from build123d import *

# Parameters (mm, degrees)
F0_R     = 75.961814
F0_R_2   = 59.912774
F1_DEPTH = 20.066
F2_R     = 7.541578
F2_R_2   = 7.528696
F2_R_3   = 6.425278
F2_R_4   = 7.130382
F2_R_5   = 7.551866
F2_R_6   = 7.528699
F2_R_7   = 7.576505
F2_R_8   = 7.567783
F3_DEPTH = 20.067
F4_SIZE  = 0.254


with BuildPart() as f1:
    # F0 (on Front) → F1 (new body)
    with BuildSketch(Plane.XZ):
        Circle(F0_R)
        Circle(F0_R_2, mode=Mode.SUBTRACT)
        Circle(F0_R_2)
        with BuildLine():
            ThreePointArc((49.361188, 15.14638), (51.061693, 7.657884), (51.632738, 0))
            ThreePointArc((51.632738, 0), (51.517245, -3.451544), (51.171281, -6.887647))
            ThreePointArc((51.171281, -6.887647), (50.183668, -12.146567), (48.657094, -17.275036))
            ThreePointArc((48.657094, -17.275036), (47.264303, -20.785219), (45.618675, -24.184213))
            ThreePointArc((45.618675, -24.184213), (40.849348, -31.579588), (34.893463, -38.057665))
            ThreePointArc((34.893463, -38.057665), (33.054915, -39.665), (31.142422, -41.183604))
            ThreePointArc((31.142422, -41.183604), (24.563545, -45.415547), (17.420865, -48.605073))
            ThreePointArc((17.420865, -48.605073), (14.606221, -49.523711), (11.74355, -50.279506))
            ThreePointArc((11.74355, -50.279506), (5.91063, -51.293314), (0, -51.632738))
            ThreePointArc((0, -51.632738), (-2.846774, -51.5542), (-5.684887, -51.318824))
            ThreePointArc((-5.684887, -51.318824), (-12.748176, -50.034225), (-19.565006, -47.782321))
            ThreePointArc((-19.565006, -47.782321), (-22.836173, -46.308194), (-25.997065, -44.61045))
            ThreePointArc((-25.997065, -44.61045), (-31.835901, -40.649908), (-37.080304, -35.930359))
            ThreePointArc((-37.080304, -35.930359), (-39.170155, -33.639837), (-41.118749, -31.228002))
            ThreePointArc((-41.118749, -31.228002), (-44.659518, -25.912682), (-47.516984, -20.200889))
            ThreePointArc((-47.516984, -20.200889), (-48.91063, -16.543575), (-50.023242, -12.791203))
            ThreePointArc((-50.023242, -12.791203), (-51.228784, -6.446033), (-51.632738, 0))
            ThreePointArc((-51.632738, 0), (-51.586992, 2.172995), (-51.449835, 4.342139))
            ThreePointArc((-51.449835, 4.342139), (-50.606227, 10.244482), (-49.087805, 16.010218))
            ThreePointArc((-49.087805, 16.010218), (-47.043655, 21.2799), (-44.435744, 26.294567))
            ThreePointArc((-44.435744, 26.294567), (-40.383346, 32.173359), (-35.558677, 37.436882))
            ThreePointArc((-35.558677, 37.436882), (-33.415529, 39.361683), (-31.168373, 41.163967))
            ThreePointArc((-31.168373, 41.163967), (-25.80143, 44.723884), (-20.033066, 47.587981))
            ThreePointArc((-20.033066, 47.587981), (-16.643542, 48.876704), (-13.171924, 49.924344))
            ThreePointArc((-13.171924, 49.924344), (-6.641125, 51.203858), (0, 51.632738))
            ThreePointArc((0, 51.632738), (2.762171, 51.558802), (5.516431, 51.337205))
            ThreePointArc((5.516431, 51.337205), (12.101384, 50.194583), (18.483581, 48.210962))
            ThreePointArc((18.483581, 48.210962), (21.402325, 46.988085), (24.240673, 45.588698))
            ThreePointArc((24.240673, 45.588698), (30.176209, 41.896731), (35.558677, 37.436882))
            ThreePointArc((35.558677, 37.436882), (37.323996, 35.677149), (39.002331, 33.83427))
            ThreePointArc((39.002331, 33.83427), (42.886907, 28.751571), (46.113144, 23.227518))
            ThreePointArc((46.113144, 23.227518), (47.907861, 19.255557), (49.361188, 15.14638))
        make_face(mode=Mode.SUBTRACT)
    extrude(amount=F1_DEPTH)

    # F2 (on Front) → F3 (cut, through all)
    with BuildSketch(Plane.XZ):
        with Locations((64.237103, 0)):
            Circle(F2_R)
        with Locations((46.261288, 43.441553)):
            Circle(F2_R_2)
        with Locations((0, 63.355938)):
            Circle(F2_R_3)
        with Locations((-46.437524, 43.794021)):
            Circle(F2_R_4)
        with Locations((-63.884638, 0)):
            Circle(F2_R_5)
        with Locations((-43.26532, -46.261288)):
            Circle(F2_R_6)
        with Locations((0, -63.532166)):
            Circle(F2_R_7)
        with Locations((42.031687, -47.142457)):
            Circle(F2_R_8)
    extrude(amount=F3_DEPTH, mode=Mode.SUBTRACT)

    # F4
    f4_edges = [f1.edges().sort_by_distance(p)[0] for p in [
        (-31.142422, 0, 41.183604),
    ]]
    chamfer(f4_edges, length=F4_SIZE)


solid = f1.part
For this review, take the finished solid that the model builds, in its own axes (mm). Round coordinates to 2 decimals unless told otherwise and drop trailing zeros. Write each loop counter-clockwise with the first axis right and the second up, starting at its lowest first coordinate (ties: lowest second). Pieces come first, ordered by that corner, then holes. Notation, with made-up numbers: M 84,-22.75 L 110,-22.75 A14 ccw 110,-3.75 Z; hole C -7.75,15 d11. An arc over 180 degrees is marked long. Write item = value, one per line. Start each with the question number.
(1) The part is to be moulded in two halves that separate along X. For faces 1 (the face through (-33.446, -10.021, 39.336)), 2 (the face through (16, 0, -50)), say which applies: +X half, -X half, draft (parallel to the pull), parting line (faces both ways), or undercut.
(2) We need section B-B (z = 2.5). Give the number of separate pieces and of enclosed holes in the cut face, then the cut area to 3 significant figures.
(3) Clearance check with flat-ended pins moving along their axes: pin 1 Ø4 at (y, z) = (-13, -16) entering from -X; pin 2 Ø1.5 at (y, z) = (-14.5, -11) entering from +X; pin 3 Ø6 at (x, y) = (8.5, -13.5) entering from +Z. State where each tip first meets the part, or that it passes through.
(4) We need section A-A (z = -58). Give the boundary of the cut face in (x, y), then the cut area to 3 significant figures.
(5) For line 1 along Z through (x, y) = (41, -1); line 2 along X through (y, z) = (-8.75, 46); line 3 along Z through (x, y) = (-42.5, -8.75), list the stretches that pass through material, from the lowest coordinate up.
Results found:
q1.face_1 = undercut
q1.face_2 = draft
q2.separate_pieces = 4
q2.enclosed_holes = 0
q2.area = 406 mm²
q3.pin_1 = -74.66
q3.pin_2 = 75.27
q3.pin_3 = 75.76
q4.outline = M -49.05,-20.07 L -5.18,-20.07 L -5.18,0 L -49.05,0 Z; M 5.18,-20.07 L 49.05,-20.07 L 49.05,0 L 5.18,0 Z
q4.area = 1,760 mm²
q5.line_1 = -63.95 to -54.64, -39.65 to -31.38, 31.38 to 38.06, 48.83 to 63.95
q5.line_2 = -60.45 to -53.22, -39.66 to -23.45, 23.45 to 39.18, 53.34 to 60.45
q5.line_3 = -62.96 to -53.75, -38.77 to -29.32, 29.32 to 37.85, 49.74 to 62.96
